Here's how the part is built. I have some questions about the finished solid (model axes, mm). A direction names the side the tool comes from. Round coordinates to 2 decimals unless told otherwise and drop trailing zeros. Loops run counter-clockwise (first coordinate to the right, second up) from the corner with the lowest first, then second, coordinate; pieces in that order, holes last. Notation, with made-up numbers: (25, 82.25) -> (72, 82.25) arc R19 ccw to (72, 110.25) -> close; hole circle Ø8 at (68.5, -3). An arc over 180 degrees is marked (long way). Use one line per item in the form item = value. Start each with the question number.
Item 1: If we section it at C-C (y = -7.25): Write out the boundary of the cut face in (x, z), then the cut area to 3 significant figures.
Item 2: If I drill on L1, parallel to Z at x = -0.15, y = 6; L2, parallel to Z at x = 0, y = -1; L3, parallel to Y at x = 0.1, z = -3, over which ranges is the centre line in solid material (lowest first)? Write a range as [from, to].
Item 3: Thinking about a two-plate mould opening in Z: for faces 3 (the face through (0.007, -14.345, -0.426)), 4 (the face through (0.007, 3.567, 10.736)), 5 (the face through (0.007, -11.262, 0.261)), 6 (the face through (0.533, -11.4, -1.1)), which applies, released by +Z, released by -Z, zero draft, split by the parting line, or undercut?
Item 4: If we section it at B-B (x = -0.2): Write out the boundary of the cut face in (y, z), then the cut area to 3 significant figures.
Item 5: For faces 1 (the face through (0.007, 3.453, -10.756)), 2 (the face through (-0.533, -11.4, -1.1)), which set-ups out of +Z, -Z, +X, -X, +Y, -Y let a thin tool reach every point of the face, with its end or its side?
Item 6: If we section it at A-A (y = -2.5): Write out the boundary of the cut face in (x, z), then the cut area to 3 significant figures.
Item 7: If we section it at D-D (z = 0): Write out the boundary of the cut face in (x, y), then the cut area to 3 significant figures.
```python
from build123d import *

# Parameters (mm, degrees)
EXTRUDE1_DEPTH = 0.5334


with BuildPart() as part:
    # Sketch1 → Extrude1 (new, symmetric)
    with BuildSketch(Plane(origin=(0, 0, 0), x_dir=(0, 0, -1), z_dir=(1, 0, 0))):
        with BuildLine():
            ThreePointArc((-12.80795, 0), (0, -11.2649), (12.80795, 0))
            ThreePointArc((12.80795, 0), (10.74595989, 3.509932598), (11.507411117, 7.508885221))
            ThreePointArc((11.507411117, 7.508885221), (11.867986747, 7.711626094), (12.229149698, 7.509933333))
            ThreePointArc((12.229149698, 7.509933333), (0, -14.351), (-12.229149698, 7.509933333))
            ThreePointArc((-12.229149698, 7.509933333), (-11.867986747, 7.711626094), (-11.507411117, 7.508885221))
            ThreePointArc((-11.507411117, 7.508885221), (-10.74595989, 3.509932598), (-12.80795, 0))
        make_face()
    extrude(amount=EXTRUDE1_DEPTH, both=True)


solid = part.part
```
Values found:
q1.outline = (-0.53, -12.39) -> (0.53, -12.39) -> (0.53, -9.36) -> (-0.53, -9.36) -> close; (-0.53, 9.36) -> (0.53, 9.36) -> (0.53, 12.39) -> (-0.53, 12.39) -> close
q1.area = 6.46 mm2
q2.L1 = [-13.04, -10.86], [10.86, 13.04]
q2.L2 = [-14.32, -12.64], [12.64, 14.32]
q2.L3 = [-14.03, -10.91]
q3.face_3 = split by the parting line
q3.face_4 = undercut
q3.face_5 = undercut
q3.face_6 = zero draft
q4.outline = (0, -12.81) arc R12.91 cw to (0, 12.81) arc R5.78 ccw to (7.51, 11.51) arc R0.42 ccw to (7.51, 12.23) arc R14.35 ccw (long way) to (7.51, -12.23) arc R0.42 ccw to (7.51, -11.51) arc R5.78 ccw to start
q4.area = 142 mm2
q5.face_1 = +X, -X
q5.face_2 = +Z, -Z, -X, +Y, -Y
q6.outline = (-0.53, -14.13) -> (0.53, -14.13) -> (0.53, -12.23) -> (-0.53, -12.23) -> close; (-0.53, 12.23) -> (0.53, 12.23) -> (0.53, 14.13) -> (-0.53, 14.13) -> close
q6.area = 4.06 mm2
q7.outline = (-0.53, -14.35) -> (0.53, -14.35) -> (0.53, -11.26) -> (-0.53, -11.26) -> close
q7.area = 3.29 mm2
